Design review of the part shown in the three views and the two pictorial views. Dimensions are in mm from the part's minimum x, y and z. A direction names the side the tool comes from. Round coordinates to 2 decimals unless told otherwise and drop trailing zeros. Loops run counter-clockwise (first coordinate to the right, second up) from the corner with the lowest first, then second, coordinate; pieces in that order, holes last. Notation, with made-up numbers: M -34.75,-33.75 L -16.75,-33.75 A14 cw -16.75,-28.75 Z; hole C -2.5,73.5 d5. An arc over 180 degrees is marked long. Answer in a Markdown table with one row per item. Add a question column.
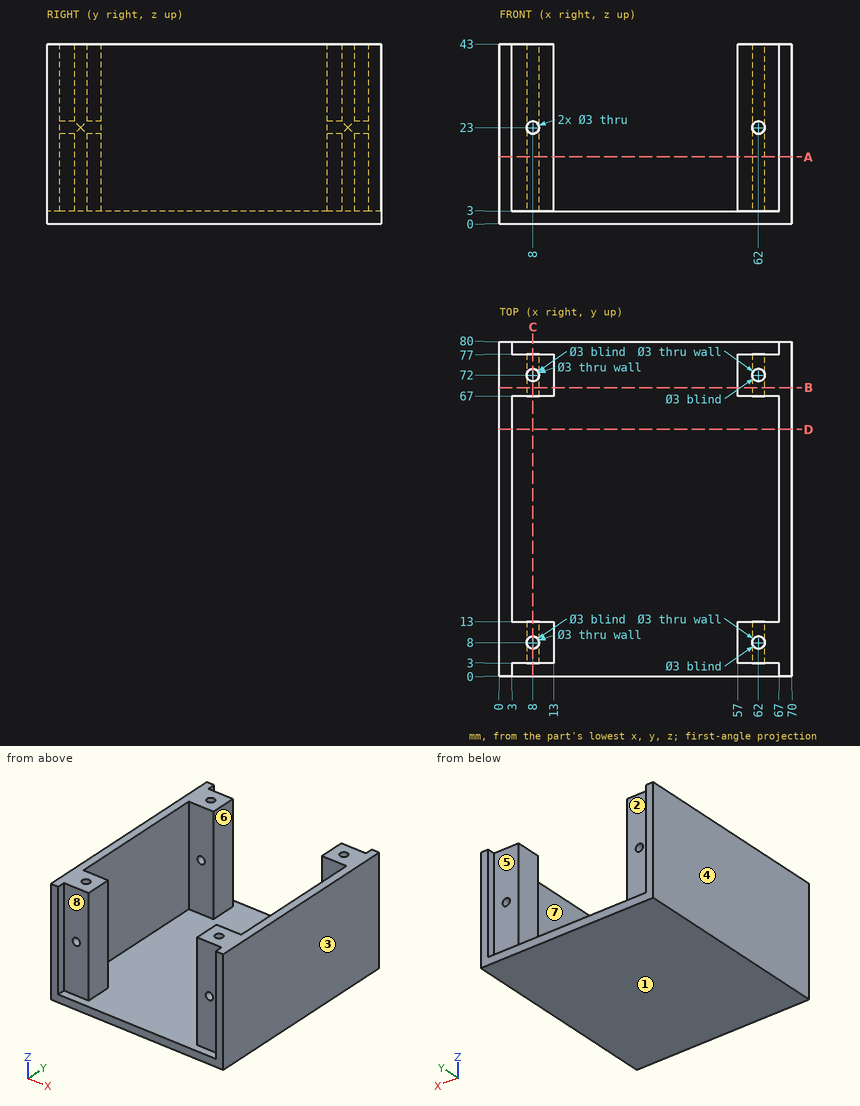
1. Take a section at C-C, the plane x = 8. State how many separate pieces and enclosed holes the cut face has, and give its area (3 significant figures).
2. Take a section at D-D, the plane y = 59. State the section outline as (x, z) points.
3. Take a section at B-B, the plane y = 69. State the section outline as (x, z) points, and give its area (3 significant figures).
4. Mouldability with a two-part tool opening along X and no side actions: class the marked faces 1, 2, 3 and 4 as released by +X, released by -X, zero draft, split by the parting line, or undercut.
5. Machinability: for the marked faces 5, 6, 7 and 8, which of the approach directions +Z, -Z, +X, -X, +Y, -Y give a long, thin tool a straight path to every point of the face, cutting with its end or side? Answer none if there is none.
6. To check wall thickness, follow probe 1 along X at (y, z) = (74, 23); probe 2 along Y at (x, z) = (62, 39); probe 3 along X at (y, z) = (43, 19.5). State the ranges of each line that lie inside material, in increasing order.
7. Take a section at A-A, the plane z = 16. State the section outline as (x, y) points.
8. For pin 1 Ø3 at (x, z) = (10, 25) entering from -Y; pin 2 Ø5 at (y, z) = (69.5, 36.5) entering from -X; pin 3 Ø1.8 at (x, y) = (62, 8) entering from +Z; pin 4 Ø5 at (x, z) = (7, 32) entering from +Y, all flat-tipped, find the tip position at first contact; note any pin that passes through.
Check sheet entries:
| question | item | result |
|---|---|---|
| 1 | separate pieces | 5 |
| 1 | enclosed holes | 0 |
| 1 | area | 758 mm^2 |
| 2 | outline | M 0,0 L 70,0 L 70,43 L 67,43 L 67,3 L 3,3 L 3,43 L 0,43 Z |
| 3 | outline | M 0,0 L 70,0 L 70,43 L 57,43 L 57,3 L 13,3 L 13,43 L 0,43 Z; hole C 8,23 d3; hole C 62,23 d3 |
| 3 | area | 1,240 mm^2 |
| 4 | face 1 | zero draft |
| 4 | face 2 | undercut |
| 4 | face 3 | released by +X |
| 4 | face 4 | released by -X |
| 5 | face 5 | +Z, +Y |
| 5 | face 6 | +Z, +Y, -Y |
| 5 | face 7 | +Z |
| 5 | face 8 | +Z, -Y |
| 6 | probe 1 | x = 0 to 6.5, 9.5 to 13, 57 to 60.5, 63.5 to 70 |
| 6 | probe 2 | y = 3 to 6.5, 9.5 to 13, 67 to 70.5, 73.5 to 77 |
| 6 | probe 3 | x = 0 to 3, 67 to 70 |
| 7 | outline | M 0,0 L 3,0 L 3,3 L 13,3 L 13,13 L 3,13 L 3,67 L 13,67 L 13,77 L 3,77 L 3,80 L 0,80 Z; M 57,3 L 67,3 L 67,0 L 70,0 L 70,80 L 67,80 L 67,77 L 57,77 L 57,67 L 67,67 L 67,13 L 57,13 Z; hole C 8,8 d3; hole C 8,72 d3; hole C 62,8 d3; hole C 62,72 d3 |
| 8 | pin 1 | stops at y = 3 |
| 8 | pin 2 | stops at x = 0 |
| 8 | pin 3 | stops at z = 3 |
| 8 | pin 4 | stops at y = 77 |
